```python
from build123d import *

# Parameters (mm, degrees)
EXTRUDE1_DEPTH     = 1.5
SKETCH2_R          = 25.4
CUT_EXTRUDE1_DEPTH = 2.5


with BuildPart() as part:
    # Sketch1 → Extrude1 (new body)
    with BuildSketch(Plane.XY):
        with BuildLine():
            Line((-338.05, 1029.967766013), (-338.05, 1077.344981378))
            ThreePointArc((-338.05, 1077.344981378), (-337.104806678, 1081.079435118), (-334.496842105, 1083.914581664))
            ThreePointArc((-334.496842105, 1083.914581664), (0, 1183.590029436), (334.496842105, 1083.914581664))
            ThreePointArc((334.496842105, 1083.914581664), (337.104806678, 1081.079435118), (338.05, 1077.344981378))
            Line((338.05, 1077.344981378), (338.05, 1029.967766013))
            Line((338.05, 1029.967766013), (-338.05, 1029.967766013))
        make_face()
    extrude(amount=EXTRUDE1_DEPTH)

    # Sketch2 → Cut-Extrude1 (cut, through all)
    with BuildSketch(Plane.XY.offset(1.5)):
        with Locations((0, 1131.567766013)):
            Circle(SKETCH2_R)
    extrude(amount=-CUT_EXTRUDE1_DEPTH, mode=Mode.SUBTRACT)


solid = part.part
```
Here's how the part is built. I have some questions about the finished solid (model axes, mm). Give positions to 0.01 mm unless a question says otherwise; leave off trailing zeros. Order: outer loops, then holes, each group sorted by start corner. A loop starts at its lowest first (then second) coordinate and runs counter-clockwise, first axis right, second up. Notation, with made-up numbers: M 16.25,33.25 L 42.25,33.25 A23 ccw 42.25,65.25 Z; hole C 41.5,50.5 d8. An arc over 180 degrees is marked long. Use a Markdown table: item, result. Add a question column.
1. Suppose I cut it at B-B (y = 1112.5). List the corners of the cut face in (x, z) for me, and give its area (3 significant figures).
2. I need wall thicknesses on probe 1 along Y at (x, z) = (0, 0.7); probe 2 along X at (y, z) = (1128.5, 1); probe 3 along Y at (x, z) = (6.5, 1.05). Which ranges of each line are inside material? Lowest first, please. Write a range as from..to.
3. Suppose I cut it at D-D (x = 198.5). List the corners of the cut face in (y, z) for me.
4. Suppose I cut it at A-A (x = 0). List the corners of the cut face in (y, z) for me.
5. If we mould it in two halves opening along X, with no side actions, what happens to faces 1 (the cylindrical face through (-4.96, 1183.57, 0.74)), 2 (the cylindrical face through (-5.506, 1106.772, 0.76)), 3 (the flat face through (5, 1091, 0))? For each: +X half, -X half, draft (parallel to the pull), parting line (faces both ways), or undercut.
6. Suppose I cut it at C-C (z = 1.25). List the corners of the cut face in (x, y) for me, and give its area (3 significant figures).
Results list:
| question | item | result |
|---|---|---|
| 1 | outline | M -286.06,0 L -16.78,0 L -16.78,1.5 L -286.06,1.5 Z; M 16.78,0 L 286.06,0 L 286.06,1.5 L 16.78,1.5 Z |
| 1 | area | 808 mm² |
| 2 | probe 1 | y = 1029.97..1106.17, 1156.97..1183.59 |
| 2 | probe 2 | x = -253.57..-25.21, 25.21..253.57 |
| 2 | probe 3 | y = 1029.97..1107.01, 1156.12..1183.56 |
| 3 | outline | M 1029.97,0 L 1150.45,0 L 1150.45,1.5 L 1029.97,1.5 Z |
| 4 | outline | M 1029.97,0 L 1106.17,0 L 1106.17,1.5 L 1029.97,1.5 Z; M 1156.97,0 L 1183.59,0 L 1183.59,1.5 L 1156.97,1.5 Z |
| 5 | face 1 | parting line |
| 5 | face 2 | undercut |
| 5 | face 3 | draft |
| 6 | outline | M -338.05,1029.97 L 338.05,1029.97 L 338.05,1077.34 A7.85 ccw 334.5,1083.91 A611.1 ccw -334.5,1083.91 A7.85 ccw -338.05,1077.34 Z; hole C 0,1131.57 d50.8 |
| 6 | area | 79,700 mm² |
